Design review of the part built by this model. Coordinates are the model's own, in mm. A direction names the side the tool comes from. Give positions to 0.01 mm unless a question says otherwise; leave off trailing zeros. Order: outer loops, then holes, each group sorted by start corner. A loop starts at its lowest first (then second) coordinate and runs counter-clockwise, first axis right, second up. Notation, with made-up numbers: (77.25, 55.5) -> (116.25, 55.5) arc R19 ccw to (116.25, 91.5) -> close; hole circle Ø11 at (18.5, -27). An arc over 180 degrees is marked (long way). Return JSON: item names as keys, results as strings.
```python
from build123d import *
from build123d.topology import SkipClean

# Parameters (mm, degrees)
CROQUIS1_R                      = 6.35
SALIENTE_EXTRUIR1_DEPTH         = 6.35
CROQUIS2_R                      = 12.5
SALIENTE_EXTRUIR2_DEPTH         = 58
CROQUIS3_R                      = 6
SALIENTE_EXTRUIR3_DEPTH         = 2
CROQUIS4_R                      = 5
SALIENTE_EXTRUIR4_DEPTH         = 11
SALIENTE_EXTRUIR5_START         = 6.35
SALIENTE_EXTRUIR5_DEPTH         = 6.35
CROQUIS7_W                      = 0.8
CROQUIS7_H                      = 0.8
CHAFL_N1_SIZE                   = 1
TALADRO_ROSCADO_M10X1_251_D     = 8.8
TALADRO_ROSCADO_M10X1_251_DEPTH = 25
TALADRO_ROSCADO_M10X1_251_TIP   = 2.643786724


with BuildPart() as part:
    # Croquis1 → Saliente-Extruir1 (new body)
    with BuildSketch(Plane.XY):
        Circle(CROQUIS1_R)
    extrude(amount=SALIENTE_EXTRUIR1_DEPTH)

    # Croquis2 → Saliente-Extruir2 (add)
    with BuildSketch(Plane.XY.offset(6.35)):
        with Locations(Location((0, 0, 0), (0, 0, 180))):
            Circle(CROQUIS2_R)
    extrude(amount=SALIENTE_EXTRUIR2_DEPTH)

    # Croquis3 → Saliente-Extruir3 (add)
    with BuildSketch(Plane.XY.offset(64.35)):
        Circle(CROQUIS3_R)
    extrude(amount=SALIENTE_EXTRUIR3_DEPTH)

    # Croquis4 → Saliente-Extruir4 (add)
    with BuildSketch(Plane.XY.offset(66.35)):
        Circle(CROQUIS4_R)
    extrude(amount=SALIENTE_EXTRUIR4_DEPTH)

    # Croquis6 → Saliente-Extruir5 (add)
    with SkipClean():  # the faces are left unmerged after this step: merging them gives an invalid solid
        with BuildSketch(Plane(origin=(0, 0, 6.35), x_dir=(-1, 0, 0), z_dir=(0, 0, -1)).offset(SALIENTE_EXTRUIR5_START)):
            with BuildLine():
                Line((-6.35, 10.76696336), (-6.35, -10.76696336))
                ThreePointArc((-6.35, -10.76696336), (0, -12.5), (6.35, -10.76696336))
                Line((6.35, -10.76696336), (6.35, 10.76696336))
                ThreePointArc((6.35, 10.76696336), (0, 12.5), (-6.35, 10.76696336))
            make_face()
        extrude(amount=-SALIENTE_EXTRUIR5_DEPTH)

    # Croquis7 → Cortar-Revolución1 (revolve, cut)
    with SkipClean():  # the faces are left unmerged after this step: merging them gives an invalid solid
        with BuildSketch(Plane(origin=(0, 0, 0), x_dir=(0, 0, -1), z_dir=(1, 0, 0)), mode=Mode.PRIVATE) as cortar_revoluci_n1_sk:
            with Locations((-74.75, 5)):
                Rectangle(CROQUIS7_W, CROQUIS7_H)
        revolve(cortar_revoluci_n1_sk.sketch.rotate(Axis((0, 0, 66.35), (0, 0, 1)), 90), axis=Axis((0, 0, 66.35), (0, 0, 1)), mode=Mode.SUBTRACT)

    # Chaflán1
    chafl_n1_edges = [part.edges().sort_by_distance(p)[0] for p in [
        (12.5, 0, 64.35),
    ]]
    chamfer(chafl_n1_edges, length=CHAFL_N1_SIZE)

    # Taladro roscado M10x1.251
    with Locations(Plane(origin=(0, 0, 0), x_dir=(-1, 0, 0), z_dir=(0, 0, -1))):
        with Locations((0, 0)):
            Hole(TALADRO_ROSCADO_M10X1_251_D / 2, depth=TALADRO_ROSCADO_M10X1_251_DEPTH)
            with Locations((0, 0, -(TALADRO_ROSCADO_M10X1_251_DEPTH + TALADRO_ROSCADO_M10X1_251_TIP / 2))):  # 118° drill point
                Cone(0, TALADRO_ROSCADO_M10X1_251_D / 2, TALADRO_ROSCADO_M10X1_251_TIP, mode=Mode.SUBTRACT)


solid = part.part
```
Item 1: For pin 1 (1.5 mm diameter, centred on x = 9.5, y = 3.5, fed in from +Z); pin 2 (1.5 mm diameter, centred on y = 7.5, z = 23, fed in from +X); pin 3 (5 mm diameter, centred on y = -4.5, z = 3, fed in from +X), all flat-tipped, find the tip position at first contact; note any pin that passes through.
Result set:
{"pin 1": "stops at z = 64.35", "pin 2": "stops at x = 10.52", "pin 3": "stops at x = 6.35"}
Item 2: Add section A-A (z = 20.5). Give the boundary of the cut face in (x, y).
Result set:
{"outline": "circle Ø25 at (0, 0); hole circle Ø8.8 at (0, 0)"}
Item 3: Add section B-B (z = 48). Give the boundary of the cut face in (x, y).
Result set:
{"outline": "circle Ø25 at (0, 0)"}
Item 4: Wall thickness on L1, parallel to X at y = 0, z = 5.75; L2, parallel to Y at x = 0, z = 11.25; L3, parallel to Z at x = -10, y = 1.5: over which ranges is each line inside the solid? List them lowest first. Write a range as [from, to].
Result set:
{"L1": "x = [-6.35, -4.4], [4.4, 6.35]", "L2": "y = [-12.5, -4.4], [4.4, 12.5]", "L3": "z = [6.35, 64.35]"}
Item 5: Mouldability with a two-part tool opening along Z and no side actions: class faces 6 (the face through (-0.729, 0.23, 27.185)), 7 (the face through (3.65, 2.8, 74.74)), 8 (the face through (0, 0, 77.35)) as released by +Z, released by -Z, zero draft, split by the parting line, or undercut.
Result set:
{"face 6": "released by -Z", "face 7": "undercut", "face 8": "released by +Z"}
Item 6: Machinability: for faces 1 (the face through (-6.35, 0, 3)), 2 (the face through (-4, 4, 66.35)), 3 (the face through (4.197, 1.322, 12.675)), 4 (the face through (-4, -3, 0)), 5 (the face through (6.35, 0, 3)), which of the approach directions +Z, -Z, +X, -X, +Y, -Y give a long, thin tool a straight path to every point of the face, cutting with its end or side? Answer none if there is none.
Result set:
{"face 1": "-Z, -X, +Y, -Y", "face 2": "+Z", "face 3": "-Z", "face 4": "-Z, +X, -X, +Y, -Y", "face 5": "-Z, +X, +Y, -Y"}
